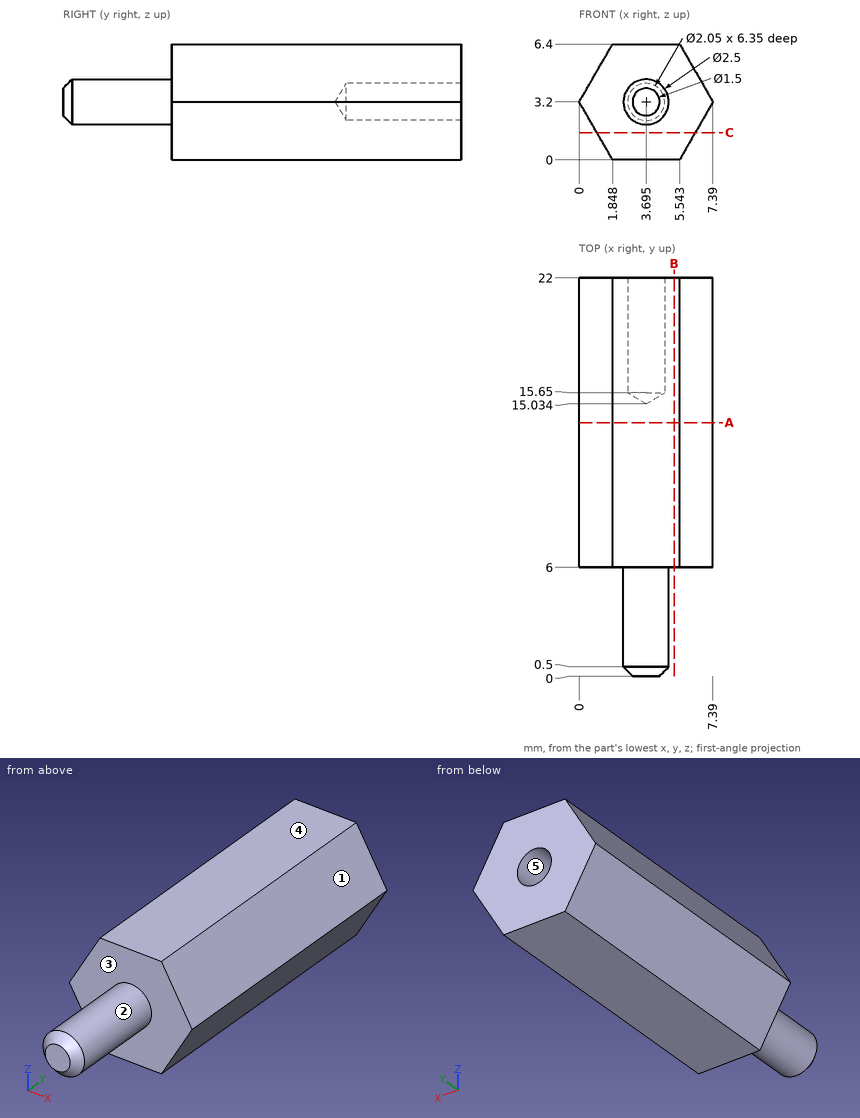
Verification items for this drawing (mm, ordinates from the low corner). A direction names the side the tool comes from. Coordinates: 2 decimals unless noted, no trailing zeros. Loops run counter-clockwise (first coordinate to the right, second up) from the corner with the lowest first, then second, coordinate; pieces in that order, holes last. Notation, with made-up numbers: (34.25, 42) - (89.25, 42) arc R37 ccw to (89.25, 79) - close; hole circle Ø8 at (69, 84.5). An arc over 180 degrees is marked (long way). Use one line per item in the form item = value. Start each with the question number.
Item 1: Section check B-B, the plane x = 5.25. Enter the section's corners in (y, z), and give its area (3 significant figures).
Item 2: Thickness scan on probe 1 along Y at (x, z) = (3.25, 4.5); probe 2 along X at (y, z) = (16, 3.5) (1 decimal); probe 3 along Z at (x, y) = (6.75, 19) (1 decimal). Record the ranges inside material, lowest first.
Item 3: Section check C-C, the plane z = 1.5. Enter the section's corners in (x, y).
Item 4: Section check A-A, the plane y = 14. Enter the section's corners in (x, z), and give its area (3 significant figures).
Item 5: Tool access check on the marked faces 1 and 2. Record the directions out of +Z, -Z, +X, -X, +Y, -Y that give a thin tool (end or side, any length) a straight path to the whole face; none if there is none.
Item 6: Mould release check, pull along Z, two halves, no side actions. Record for the marked faces 3, 4 and 5: +Z half, -Z half, draft (parallel to the pull), parting line (faces both ways), or undercut.
Computed:
q1.outline = (6, 0) - (22, 0) - (22, 6.4) - (6, 6.4) - close
q1.area = 102 mm2
q2.probe_1 = 6 to 22
q2.probe_2 = 0.2 to 2.7, 4.7 to 7.2
q2.probe_3 = 2.1 to 4.3
q3.outline = (0.98, 6) - (6.41, 6) - (6.41, 22) - (0.98, 22) - close
q4.outline = (0, 3.2) - (1.85, 0) - (5.54, 0) - (7.39, 3.2) - (5.54, 6.4) - (1.85, 6.4) - close
q4.area = 35.5 mm2
q5.face_1 = +Z, +X, +Y, -Y
q5.face_2 = -Y
q6.face_3 = draft
q6.face_4 = +Z half
q6.face_5 = undercut
